The listing builds one solid part. Answer for the finished solid, in the listing's coordinates (mm). A direction names the side the tool comes from. Coordinates: 2 decimals unless noted, no trailing zeros. Write each loop counter-clockwise with the first axis right and the second up, starting at its lowest first coordinate (ties: lowest second). Pieces come first, ordered by that corner, then holes.
from build123d import *

# Parameters (mm, degrees)
F1_DEPTH = 139.7
F0_W     = 50.8
F0_H     = 24.8791221529
F2_DEPTH = 63.5
F3_R     = 25.4
F5_D     = 19.05
F6_D     = 31.75
F6_DEPTH = 25.4
F6_TIP   = 9.5386623271
F8_D     = 12.7


with BuildPart() as f1:
    # F0 (on Right) → F1 (new body)
    with BuildSketch(Plane.YZ):
        with BuildLine():
            Line((0, 63.5), (0, 31.75))
            Line((0, 31.75), (50.8, 63.5))
            Line((50.8, 63.5), (50.8, 101.6))
            Line((50.8, 101.6), (25.4, 101.6))
            ThreePointArc((25.4, 101.6), (7.4394877579, 94.1605122421), (0, 76.2))
            Line((0, 76.2), (0, 63.5))
        make_face()
    extrude(amount=F1_DEPTH)

    # F0 (on Right) → F2 (join)
    with BuildSketch(Plane.YZ):
        Polygon((0, 31.75), (0, 24.8791221529), (50.8, 24.8791221529), (50.8, 63.5), align=None)
        with Locations((25.4, 12.4395610765)):
            Rectangle(F0_W, F0_H)
    extrude(amount=F2_DEPTH)

    # F3
    f3_edges = [f1.edges().sort_by_distance(p)[0] for p in [
        (63.5, 25.4, 0),
    ]]
    fillet(f3_edges, radius=F3_R)

    # F5 (through all)
    with Locations(Plane(origin=(0, 50.8, 0), x_dir=(-1, 0, 0), z_dir=(0, 1, 0))):
        with Locations((-19.05, 25.4)):
            Hole(F5_D / 2)

    # F6
    with Locations(Plane(origin=(0, 50.8, 0), x_dir=(-1, 0, 0), z_dir=(0, 1, 0))):
        with Locations((-19.05, 25.4)):
            Hole(F6_D / 2, depth=F6_DEPTH)
            with Locations((0, 0, -(F6_DEPTH + F6_TIP / 2))):  # 118° drill point
                Cone(0, F6_D / 2, F6_TIP, mode=Mode.SUBTRACT)

    # F8 (through all)
    with Locations(Plane.XY.offset(101.6)):
        with Locations((114.3, 38.1)):
            Hole(F8_D / 2)


solid = f1.part
1. Find the intervals of material crossed by L1, parallel to X at y = 38, z = 84; L2, parallel to Z at x = 19.05, y = 44.5 (3 decimals); L3, parallel to X at y = 39.5, z = 17.5, in increasing order.
Results found:
L1: x = 0 to 107.95, 120.65 to 139.7
L2: z = 0 to 9.525, 41.275 to 101.6
L3: x = 0 to 5.28, 32.82 to 62.24
2. Section C-C on z = 71.5 is taken. Give the vertices of the cut face in (x, y), then the cut area to 3 significant figures.
Results found:
outline: (0, 0) - (139.7, 0) - (139.7, 50.8) - (0, 50.8) - close; hole circle Ø12.7 at (114.3, 38.1)
area: 6,970 mm2
3. A tool of negligible diameter and unlimited length cuts with its end or side. For faces 1 (the cylindrical face through (115.68, 31.9, 76.25)), 2 (the cylindrical face through (7.35, 37.92, 36.13)), 3 (the flat face through (63.5, 31, 40)), from which of +Z, -Z, +X, -X, +Y, -Y can it reach the whole face along a straight path? Write none if from no direction.
Results found:
face 1: +Z, -Z
face 2: +Y
face 3: -Z, +X, +Y
4. Section B-B on x = 19.05 is taken. Give the vertices of the cut face in (y, z) (3 decimals).
Results found:
outline: (0, 0) - (50.8, 0) - (50.8, 9.525) - (25.4, 9.525) - (21.585, 15.875) - (0, 15.875) - close; (0, 34.925) - (21.585, 34.925) - (25.4, 41.275) - (50.8, 41.275) - (50.8, 101.6) - (25.4, 101.6) arc R25.4 ccw to (0, 76.2) - close
5. For a pull along Z with two mould halves and no side action, classify faces 4 (the conical face through (13.716, 21.823, 33.766)), 5 (the cylindrical face through (68.87, 7.64, 94.36)), 6 (the flat face through (101.07, 25.04, 47.4)) as pulls with the +Z half, pulls with the -Z half, needs draft (parallel to the pull), parting line crosses it, or undercut.
Results found:
face 4: undercut
face 5: pulls with the +Z half
face 6: pulls with the -Z half
6. Section A-A on y = 38.1 is taken. State how many separate pieces and enclosed holes the cut face has, then the cut area to 3 significant figures.
Results found:
separate pieces: 2
enclosed holes: 1
area: 8,440 mm2
7. A flat-ended cylindrical pin translates along its axis: P1, Ø2, axis at x = 96, y = 6.5, coming from the -Z side. Find the tip coordinate at first contact, or state that the pin passes through.
Results found:
P1: stops at z = 35.19
8. Section D-D on y = 14 is taken. Give the vertices of the cut face in (x, z) (3 decimals), then the cut area to 3 significant figures.
Results found:
outline: (0, 0) - (38.1, 0) arc R25.4 ccw to (63.5, 25.4) - (63.5, 40.5) - (139.7, 40.5) - (139.7, 98.898) - (0, 98.898) - close; hole circle Ø19.05 at (19.05, 25.4)
area: 10,300 mm2
